Build history of the part. All positions in model axes, mm. A direction names the side the tool comes from. Round coordinates to 2 decimals unless told otherwise and drop trailing zeros. Write each loop counter-clockwise with the first axis right and the second up, starting at its lowest first coordinate (ties: lowest second). Pieces come first, ordered by that corner, then holes. Notation, with made-up numbers: M 84,-23 L 94,-23 A10 cw 94,-5 Z; hole C 4,67.25 d7. An arc over 180 degrees is marked long. Use a Markdown table: item, result.
Autodesk Inventor part; units mm, degrees
ref_plane "YZ Plane" through (0, 0, 0) normal (1, 0, 0) x (0, 1, 0)
ref_plane "XZ Plane" through (0, 0, 0) normal (0, 1, 0) x (-1, 0, 0)
ref_plane "XY Plane" through (0, 0, 0) normal (0, 0, 1) x (1, 0, 0)
sketch "Sketch1" plane through (0, 0, 0) normal (0, 0, 1) x (1, 0, 0)
  line L0 (0, 0) -> (19, 0)
  line L1 (19, 0) -> (19, 9)
  line L2 (19, 9) -> (0, 9)
  line L3 (0, 9) -> (0, 0)
  point P0 (9.5, 9)
  dimension "d0" = 19
  dimension "d1" = 9
extrude "Extrusion1" add sketch "Sketch1" along normal blind 3
sketch "Sketch10" plane through (0, 0, 0) normal (-1, 0, 0) x (0, 0, 1)
  line L0 (0, 0) -> (3, 0)
  line L1 (3, 9) -> (3, 0)
  line L2 (3, 0) -> (2, 0)
  line L3 (2, 0) -> (2, 6)
  line L4 (2, 6) -> (3, 6)
  line L5 (3, 6) -> (3, 0)
  line L6 (3, 0) -> (2, 1)
  line L7 (3, 0) -> (4.4142, 0) construction
  line L8 (2, 1) -> (3, 2)
  line L9 (3, 0) -> (3, 9)
  line L10 (3, 2) -> (2, 3)
  line L11 (2, 3) -> (3, 4)
  line L12 (2, 5) -> (3, 4)
  line L13 (2, 5) -> (3, 5)
  dimension "d23" = 1
  dimension "d24" = 6
  dimension "d25" = 135
  dimension "d26" = 90
extrude "Extrusion8" cut sketch "Sketch10" against normal up to next contours L6 L8 L1 | L10 L11 L1 | L12 L13 L1 | L3 L4 L1 L13
sketch "Sketch11" plane through (0, 0, 0) normal (0, -1, 0) x (1, 0, 0)
  line L0 (0, 3) -> (19, 3)
  line L1 (0, 3) -> (19, 3)
  line L2 (19, 3) -> (19, 2)
  line L3 (19, 2) -> (8.5, 2)
  line L4 (0, 2) -> (0, 3)
  line L5 (0, 3) -> (0, 2)
  line L6 (0, 3) -> (1.4142, 3) construction
  line L7 (19, 3) -> (0, 3)
  line L8 (9.5, 3) -> (8.5, 2)
  line L9 (9.5, 3) -> (10.9142, 3) construction
  line L10 (10.5, 2) -> (8.5, 2)
  line L11 (9.5, 3) -> (10.5, 2)
  line L12 (10.5, 2) -> (8.5, 2)
  line L13 (8.5, 2) -> (0, 2)
  line L14 (7.5, 3) -> (8.5, 2)
  line L15 (8.5, 2) -> (6.5, 2)
  line L16 (7.5, 3) -> (6.5, 2)
  line L17 (5.5, 3) -> (6.5, 2)
  line L18 (6.5, 2) -> (4.5, 2)
  line L19 (5.5, 3) -> (4.5, 2)
  line L20 (3.5, 3) -> (4.5, 2)
  line L21 (4.5, 2) -> (2.5, 2)
  line L22 (3.5, 3) -> (2.5, 2)
  line L23 (12.5, 2) -> (10.5, 2)
  line L24 (11.5, 3) -> (12.5, 2)
  line L25 (11.5, 3) -> (10.5, 2)
  line L26 (14.5, 2) -> (12.5, 2)
  line L27 (13.5, 3) -> (14.5, 2)
  line L28 (13.5, 3) -> (12.5, 2)
  line L29 (16.5, 2) -> (14.5, 2)
  line L30 (15.5, 3) -> (16.5, 2)
  line L31 (15.5, 3) -> (14.5, 2)
  point P0 (0, 0)
  dimension "d30" = 135
  dimension "d33" = 2
  dimension "d40" = 2
extrude "Extrusion9" cut sketch "Sketch11" against normal blind 6 contours L0 L22 L13 L4 | L0 L19 L20 | L0 L16 L17 | L0 L8 L14 | L0 L25 L11 | L0 L28 L24 | L0 L31 L27 | L0 L2 L3 L30
sketch "Sketch12" plane through (0, 0, 3) normal (0, 0, 1) x (1, 0, 0)
  line L0 (19, 9) -> (0, 9)
  line L1 (11.5494, 5.9) -> (7.4494, 5.9)
  line L2 (7.4494, 5.9) -> (7.4494, 8.1)
  line L3 (7.4494, 8.1) -> (11.5494, 8.1)
  line L4 (11.5494, 8.1) -> (11.5494, 5.9)
  line L5 (11.5494, 5.9) -> (7.4494, 8.1) construction
  line L6 (7.4494, 5.9) -> (11.5494, 8.1) construction
  line L7 (10.5994, 7.2) -> (8.3994, 7.2)
  line L8 (8.3994, 7.2) -> (8.3994, 9)
  line L9 (8.3994, 9) -> (10.5994, 9)
  line L10 (10.5994, 9) -> (10.5994, 7.2)
  line L11 (10.5994, 7.2) -> (8.3994, 9) construction
  line L12 (8.3994, 7.2) -> (10.5994, 9) construction
  point P0 (0, 0)
  point P1 (9.4994, 7)
  point P2 (9.4994, 8.1)
  dimension "d47" = 2
  dimension "d48" = 4.1
  dimension "d49" = 2.2
  dimension "d50" = 2.2
extrude "Extrusion10" cut sketch "Sketch12" against normal up to next
sketch "Sketch13" plane through (0, 0, 0) normal (0, 0, -1) x (-1, 0, 0)
  line L0 (-8.3994, 9) -> (-8.3994, 8.1)
  line L1 (-8.3994, 8.1) -> (-7.4494, 8.1)
  line L2 (-7.4494, 8.1) -> (-7.4494, 5.9)
  line L3 (-7.4494, 5.9) -> (-11.5494, 5.9)
  line L4 (-11.5494, 5.9) -> (-11.5494, 8.1)
  line L5 (-11.5494, 8.1) -> (-10.5994, 8.1)
  line L6 (-10.5994, 8.1) -> (-10.5994, 9)
  line L7 (-19, 9) -> (-10.5994, 9)
  line L8 (-19, 0) -> (-19, 9)
  line L9 (0, 0) -> (-19, 0)
  line L10 (0, 9) -> (0, 0)
  line L11 (-8.3994, 9) -> (0, 9)
  line L12 (-10.5, 3) -> (-8.5, 3)
  line L13 (-1, 5) -> (-18, 5)
  line L14 (-18, 5) -> (-18, 1)
  line L15 (-18, 1) -> (-1, 1)
  line L16 (-1, 1) -> (-1, 5)
  line L17 (-1, 5) -> (-18, 1) construction
  line L18 (-18, 5) -> (-1, 1) construction
  point P0 (-9.5, 3)
  dimension "d53" = 17
  dimension "d54" = 4
extrude "Extrusion11" cut sketch "Sketch13" against normal blind 1 contours L16 L15 L14 L13
sketch "Sketch14" plane through (0, 0, 2) normal (0, 0, 1) x (1, 0, 0)
  line L0 (6.4994, 5) -> (12.4994, 5)
  line L1 (12.4994, 5) -> (12.4994, 6)
  line L2 (12.4994, 6) -> (6.4994, 6)
  line L3 (6.4994, 6) -> (6.4994, 5)
  line L4 (6.4994, 5) -> (12.4994, 6) construction
  line L5 (12.4994, 5) -> (6.4994, 6) construction
  line L6 (19, 9) -> (10.5994, 9)
  point P0 (0, 0)
  point P1 (9.4994, 5.5)
  dimension "d57" = 6
  dimension "d58" = 1
  dimension "d59" = 3.5
extrude "Extrusion12" add sketch "Sketch14" along normal blind 1
chamfer "Chamfer1" distance 0.5 angle 45 1 edges at (9.4994, 5, 3)
sketch "WeightSection-5mm" plane through (0, 0, 0) normal (-1, 0, 0) x (0, 0, 1)
  line L0 (0, 5) -> (1, 5)
  line L1 (1, 5) -> (1, 1)
  line L2 (0, 1) -> (1, 1)
  circle A0 centre (-1.5334, 3) radius 2.5
  point P0 (0, 0)
  dimension "d65" = 5
properties part number "Clamp-part2(moving)-Base9x19mm."
Q1. Cut at B-B on x = 16.25. Give the cut face in (y, z), and give its area (3 significant figures).
Response values:
| item | result |
|---|---|
| outline | M 0,0 L 1,0 L 1,1 L 5,1 L 5,0 L 9,0 L 9,3 L 6,3 L 6,2 L 5,2 L 4.75,2.25 L 3.25,2.25 L 3,2 L 2.75,2.25 L 1.25,2.25 L 1,2 L 0.75,2.25 L 0,2.25 Z |
| area | 18.1 mm2 |
Q2. Which spindle directions (+Z, -Z, +X, -X, +Y, -Y) get a long thin tool onto all of the face, cutting with end or side? Do faces 4 (the flat face through (15.7, 6, 2.5)), 5 (the flat face through (2.9, 2, 2.4)), 6 (the flat face through (4.1, 4, 2.4)), 7 (the flat face through (8, 8.1, 2)). Say none if no direction does.
Response values:
| item | result |
|---|---|
| face 4 | +Z, +X |
| face 5 | +Z, -X, -Y |
| face 6 | +Z, -Y |
| face 7 | +Z, -Z |
Q3. Cut at C-C on z = 0.3. Give the cut face in (x, y), and give its area (3 significant figures).
Response values:
| item | result |
|---|---|
| outline | M 0,0 L 19,0 L 19,9 L 10.6,9 L 10.6,8.1 L 11.55,8.1 L 11.55,5.9 L 7.45,5.9 L 7.45,8.1 L 8.4,8.1 L 8.4,9 L 0,9 Z; hole M 1,1 L 18,1 L 18,5 L 1,5 Z |
| area | 92.0 mm2 |
Q4. Cut at D-D on z = 1.8. Give the cut face in (x, y), and give its area (3 significant figures).
Response values:
| item | result |
|---|---|
| outline | M 0,0 L 19,0 L 19,9 L 10.6,9 L 10.6,8.1 L 11.55,8.1 L 11.55,5.9 L 7.45,5.9 L 7.45,8.1 L 8.4,8.1 L 8.4,9 L 0,9 Z |
| area | 160 mm2 |
Q5. Drill centre lines: L1, parallel to X at y = 6.25, z = 2.3; L2, parallel to Y at x = 11.5, z = 2.7; L3, parallel to Y at x = 10.75, z = 2.35. Where is each one in solid material? Low to high.
Response values:
| item | result |
|---|---|
| L1 | x = 0 to 7.45, 11.55 to 19 |
| L2 | y = 0 to 0.3, 1.7 to 2.3, 3.7 to 4.3, 5.2 to 6, 8.1 to 9 |
| L3 | y = 5 to 6, 8.1 to 9 |
Q6. Cut at A-A on y = 7.5. Give the cut face in (x, z), and give its area (3 significant figures).
Response values:
| item | result |
|---|---|
| outline | M 0,0 L 7.45,0 L 7.45,3 L 0,3 Z; M 11.55,0 L 19,0 L 19,3 L 11.55,3 Z |
| area | 44.7 mm2 |
Q7. Drop flat-ended pins along their axis: P1, Ø0.5, axis at x = 10, z = 2.5, coming from the +Y side; P2, Ø3, axis at x = 5.5, y = 3, coming from the -Z side; P3, Ø1.8, axis at x = 2.5, y = 4, coming from the +Z side. Give the stop position or say it passes through.
Response values:
| item | result |
|---|---|
| P1 | stops at y = 6 |
| P2 | stops at z = 1 |
| P3 | stops at z = 2.9 |
Q8. Two-plate mould, pull along Y, no slides. Class faces 1 (the flat face through (4.9, 4, 2.4)), 2 (the flat face through (5.5, 1.4, 2.4)), 3 (the flat face through (4, 9, 1)): +Y half, -Y half, draft (parallel to the pull), parting line (faces both ways), or undercut.
Response values:
| item | result |
|---|---|
| face 1 | draft |
| face 2 | undercut |
| face 3 | +Y half |
